from build123d import *

# Parameters (mm, degrees)
F0_W     = 60
F0_H     = 67.5
F1_DEPTH = 15
F5_DEPTH = 7
F7_DEPTH = 4


with BuildPart() as f1:
    # F0 (on Top) → F1 (new body)
    with BuildSketch(Plane.XY):
        with Locations((-30, 33.75)):
            Rectangle(F0_W, F0_H)
        Polygon((60, 67.5), (0, 67.5), (0, 0), (5.9781013988, 0), (60, 0), align=None)
        with Locations((-30, -33.75)):
            Rectangle(F0_W, F0_H)
        Polygon((5.9781013988, 0), (0, 0), (0, -67.5), (60, -67.5), (60, 0), align=None)
    extrude(amount=F1_DEPTH)

    # F4 (on face) → F5 (join)
    with BuildSketch(Plane.XY.offset(15)):
        with BuildLine():
            Line((-60, 0), (-60, -38.0529202521))
            ThreePointArc((-60, -38.0529202521), (-49.5105953574, -51.0904314292), (-33.6693982898, -56.4812368343))
            ThreePointArc((-33.6693982898, -56.4812368343), (-15.3376274344, -57.4161028449), (0, -67.5))
            ThreePointArc((0, -67.5), (12.9433258402, -58.7363497884), (28.410895604, -56.4812368343))
            ThreePointArc((28.410895604, -56.4812368343), (47.3381804243, -52.6370871063), (60, -38.0529202521))
            Line((60, -38.0529202521), (60, 67.5))
            Line((60, 67.5), (-60, 67.5))
            Line((-60, 67.5), (-60, 0))
        make_face()
    extrude(amount=F5_DEPTH)

    # F6 (on face) → F7 (join)
    with BuildSketch(Plane.XY.offset(22)):
        with BuildLine():
            add(Edge.make_bspline(
                [(-60, -14.1512239352), (-59.0293889919, -13.7585961079), (-56.6236997139, -12.7854559454), (-49.0504631043, -12.3499323054), (-41.4676376213, -14.4143905876), (-37.310563853, -17.3961414407), (-31.6113048526, -13.7340453951), (-24.3327976689, -12.9655279158), (-16.730226682, -15.1518072312), (-11.848805959, -17.9023620476), (-6.6941574417, -19.2385563279), (-2.0295442031, -18.0148753376), (-0.0189397587, -16.5628165681), (0.1118455984, -16.2781241236)],
                knots=[0, 0, 0, 0, 0.0705560873, 0.1748754354, 0.2822587754, 0.3622366871, 0.454972104, 0.5582662803, 0.6642203819, 0.7542834332, 0.8403652981, 0.925033899, 0.9832160145, 0.9832160145, 0.9832160145, 0.9832160145], degree=3))
            Line((-60, -14.1512239352), (-60, -19.8548957705))
            add(Edge.make_bspline(
                [(-60, -19.8548957705), (-58.7257888093, -19.1436585072), (-55.8955547979, -17.5638827938), (-48.9702862444, -17.3858195386), (-42.4680056618, -19.1850661251), (-37.463020039, -22.1911615113), (-30.3087693341, -18.677386885), (-24.871896529, -17.4062862995), (-16.9093310744, -19.8677835147), (-12.7943307223, -21.7909091619), (-6.3861561614, -24.228006265), (-2.0676772483, -22.3592450119), (0.1470434485, -21.4008556559)],
                knots=[0, 0, 0, 0, 0.0855559678, 0.190033969, 0.2947188809, 0.3878397063, 0.4961411128, 0.5926967688, 0.7053736836, 0.7934295061, 0.8940608586, 1, 1, 1, 1], degree=3))
            Line((0.1470434485, -21.4008556559), (0.1118455984, -16.2781241236))
        make_face()
        with BuildLine():
            add(Edge.make_bspline(
                [(-60, -27.6262178335), (-58.6908579139, -27.0610454374), (-55.7423438806, -25.7881364393), (-48.6094061642, -23.7011458379), (-36.3948711424, -30.1574496981), (-26.1879734271, -21.9651117607), (-14.2133970996, -28.0543249168), (-5.5258287766, -29.9499942904), (-1.5805656805, -28.3459920046), (0.1898173795, -27.6262178335)],
                knots=[0, 0, 0, 0, 0.1030829205, 0.2321684107, 0.4040915702, 0.5670970962, 0.7386692977, 0.882731408, 1, 1, 1, 1], degree=3))
            Line((-60, -27.6262178335), (-60, -33.2923606038))
            add(Edge.make_bspline(
                [(-60, -33.2923606038), (-56.3803265128, -31.5433703048), (-48.9851936137, -27.9701154943), (-36.844872956, -36.1289431011), (-25.2372817337, -26.9445755845), (-14.8016717458, -33.2381042089), (-4.5983556928, -34.4314814953), (-1.2173570397, -32.2734966719), (0.2154648118, -31.358971667)],
                knots=[0, 0, 0, 0, 0.1761592769, 0.3599002143, 0.5422376138, 0.7167772716, 0.879974009, 1, 1, 1, 1], degree=3))
            Line((0.2154648118, -31.358971667), (0.1898173795, -27.6262178335))
        make_face()
    extrude(amount=F7_DEPTH)


solid = f1.part
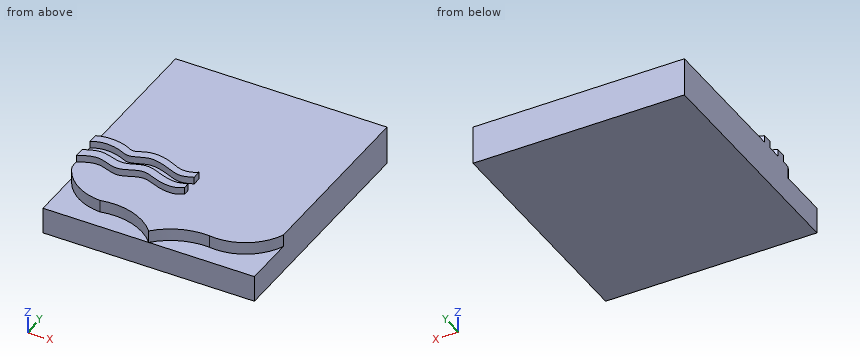
Input: part model. Units: mm. Frame: model coordinates. Round coordinates to 2 decimals unless told otherwise and drop trailing zeros. Order: outer loops, then holes, each group sorted by start corner. A loop starts at its lowest first (then second) coordinate and runs counter-clockwise, first axis right, second up. Notation, with made-up numbers: (-6.75, 13) - (1.25, 13) arc R14 ccw to (1.25, 19) - close; hole circle Ø6 at (53.5, -38). An arc over 180 degrees is marked (long way). Answer as a JSON object with one key per item and string values. Group by question number.
(1) Cut plane B-B (y = -54). Return loops of the section in (x, z), then the cut area to 3 significant figures.
(2) Cut plane A-A (z = 18.25). Return loops of the section in (x, y), then the cut area to 3 significant figures.
(3) Pin query (flat end, axial travel): P1, Ø2, axis at x = 32, y = -14, coming from the +Z side. Return the tip coordinate at first contact, or that it passes through.
(4) Cut plane C-C (x = 25). Return loops of the section in (y, z), then the cut area to 3 significant figures.
(5) Material intervals for probe 1 along Z at (x, y) = (-27.5, -49); probe 2 along Y at (x, z) = (25.5, 15.5); probe 3 along Y at (x, z) = (-49.5, 23.75), sorted ascending. Write a range as from..to.
(6) Cut plane D-D (y = -6.5). Return loops of the section in (x, z), then the cut area to 3 significant figures.
Here are the results:
{
 "1": {"outline": "(-60, 0) - (60, 0) - (60, 15) - (44.71, 15) - (44.71, 22) - (-44.33, 22) - (-44.33, 15) - (-60, 15) - close", "area": "2,420 mm^2"},
 "2": {"outline": "(-60, -38.05) arc R30 ccw to (-33.67, -56.48) arc R35 cw to (0, -67.5) arc R35 cw to (28.41, -56.48) arc R30 ccw to (60, -38.05) - (60, 67.5) - (-60, 67.5) - close", "area": "14,800 mm^2"},
 "3": {"P1": "stops at z = 22"},
 "4": {"outline": "(-67.5, 0) - (67.5, 0) - (67.5, 22) - (-56.37, 22) - (-56.37, 15) - (-67.5, 15) - close", "area": "2,890 mm^2"},
 "5": {"probe 1": "z = 0..22", "probe 2": "y = -56.37..67.5", "probe 3": "y = -30.16..-24.91, -17.68..-12.77"},
 "6": {"outline": "(-60, 0) - (60, 0) - (60, 22) - (-60, 22) - close", "area": "2,640 mm^2"}
}
